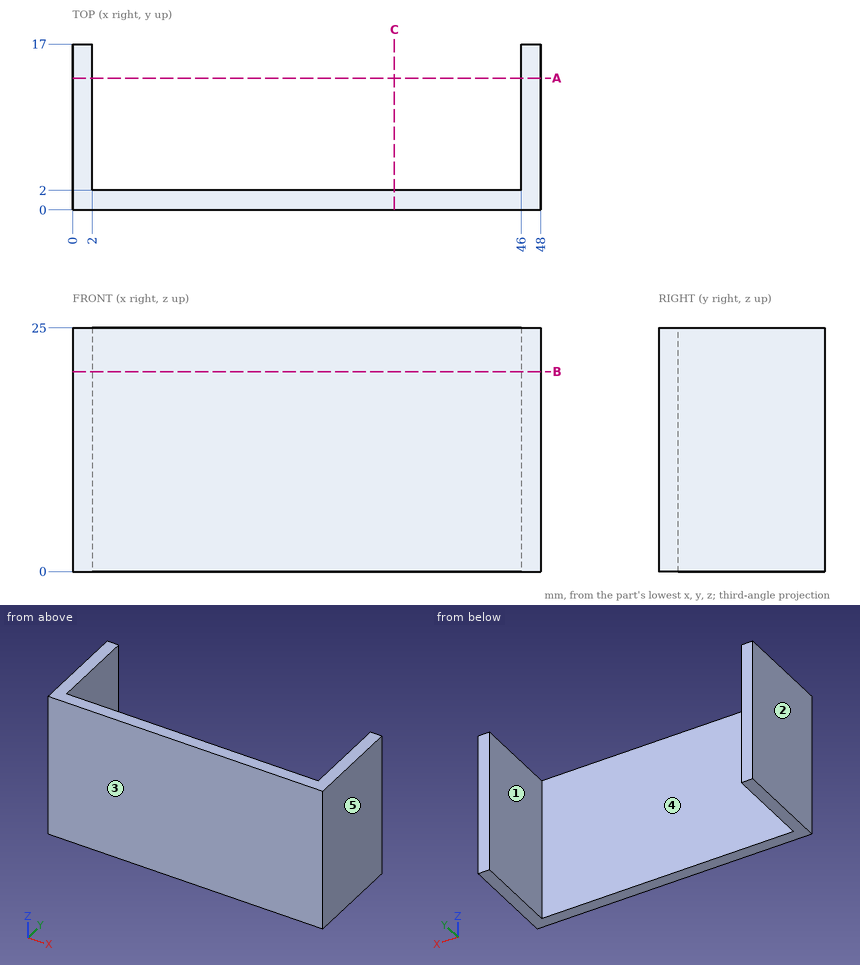
Input: dimensioned drawing with shaded views. Units: mm. Origin: part minimum x, y, z. A direction names the side the tool comes from. Coordinates: 2 decimals unless noted, no trailing zeros. Order: outer loops, then holes, each group sorted by start corner. A loop starts at its lowest first (then second) coordinate and runs counter-clockwise, first axis right, second up.
Item 1: Section query B-B (z = 20.5). Output: boundary loops of the cut face in (x, y).
Answer:
outline: (0, 0) - (48, 0) - (48, 17) - (46, 17) - (46, 2) - (2, 2) - (2, 17) - (0, 17) - close
Item 2: Contact query for a flat-ended pin moving along its axis: P1, Ø2, axis at x = 14.5, z = 3, coming from the +Y side. Output: stop coordinate, or through.
Answer:
P1: stops at y = 2
Item 3: Section query A-A (y = 13.5). Output: boundary loops of the cut face in (x, z), then the cut area to 3 significant figures.
Answer:
outline: (0, 0) - (2, 0) - (2, 25) - (0, 25) - close; (46, 0) - (48, 0) - (48, 25) - (46, 25) - close
area: 100 mm2
Item 4: Material intervals for line 1 along X through (y, z) = (15.5, 3.25); line 2 along Y through (x, z) = (3, 1.5), sorted ascending.
Answer:
line 1: x = 0 to 2, 46 to 48
line 2: y = 0 to 2
Item 5: Section query C-C (x = 33). Output: boundary loops of the cut face in (y, z), then the cut area to 3 significant figures.
Answer:
outline: (0, 0) - (2, 0) - (2, 25) - (0, 25) - close
area: 50.0 mm2
Item 6: Access query for the marked faces 1 and 2. Directions: +Z, -Z, +X, -X, +Y, -Y. A direction counts if a zero-diameter tool reaches every point of the face in a straight line with its end or side. Return the directions, or none.
Answer:
face 1: +Z, -Z, +Y
face 2: +Z, -Z, -X, +Y, -Y
Item 7: Draft query along X for the marked faces 3, 4 and 5. Return one class per face: released by +X, released by -X, zero draft, split by the parting line, or undercut.
Answer:
face 3: zero draft
face 4: undercut
face 5: released by +X
